Model file for the job. Use its own axes, mm. A direction names the side the tool comes from. Round coordinates to 2 decimals unless told otherwise and drop trailing zeros. Loops run counter-clockwise (first coordinate to the right, second up) from the corner with the lowest first, then second, coordinate; pieces in that order, holes last. Notation, with made-up numbers: M -31,22.5 L 2,22.5 A13 cw 2,38.5 Z; hole C 18,40.25 d2. An arc over 180 degrees is marked long. Use a Markdown table: item, result. Add a question column.
Item 1: Pin check, flat tips, straight feed: P1, Ø1, axis at x = 19.5, y = 10, coming from the -Z side; P2, Ø8.5, axis at x = -25.5, z = 47, coming from the -Y side; P3, Ø0.9, axis at x = -37.5, y = 5.5, coming from the -Z side. Stop position of each tip, or through.
Item 2: Tool access for faces 5 (the cylindrical face through (-16.14, 13.25, 51.03)), 6 (the flat face through (0, 5.25, 48)), 7 (the flat face through (-1, 16, 46)), 8 (the flat face through (-37, -2.95, 29)), 9 (the flat face through (37, 5, 21.5)): list every direction of +Z, -Z, +X, -X, +Y, -Y with a clear straight run to the whole face (end or side of a thin tool).
Item 3: Two-plate mould, pull along X, no slides. Class faces 1 (the flat face through (42, 23, 34.244)), 2 (the flat face through (43, 13, 38)), 3 (the flat face through (1, 16, 46)), 4 (the cylindrical face through (-38.19, 6.16, 17.95)): +X half, -X half, draft (parallel to the pull), parting line (faces both ways), or undercut.
Item 4: Saw through at D-D on z = 46. Give the number of separate pieces and of enclosed holes in the cut face, then the cut area to 3 significant figures.
Item 5: Saw through at C-C on x = 37. Write the cut outline in (y, z), then the cut area to 3 significant figures.
Item 6: Saw through at A-A on z = 19. Write the cut outline in (x, y), then the cut area to 3 significant figures.
Item 7: Wall check: L1, parallel to X at y = 5, z = 18; L2, parallel to Y at x = 37, z = 17.75; L3, parallel to X at y = 8, z = 27. Give the ranges that are in metal, low to high. Write a range as from..to.
Item 8: Saw through at B-B on z = 40. Write the cut outline in (x, y), then the cut area to 3 significant figures.
```python
from build123d import *

# Parameters (mm, degrees)
F0_W          = 12
F0_H          = 16.5
F0_R          = 1.6
F1_DEPTH      = 17.5
F5_W          = 12
F5_H          = 16.5
F6_DEPTH      = 3
F2_W          = 12
F2_H          = 16.4
F7_DEPTH      = 35.5
F7_DEPTH_BACK = 3
F11_W         = 50
F11_H         = 5.5
F12_DEPTH     = 90
F14_DEPTH     = 10
F15_R         = 1.5
F16_DEPTH     = 7
F17_R         = 8
F18_DEPTH     = 15
F22_R         = 8
F22_R_2       = 6
F23_DEPTH     = 6
F25_DEPTH     = 25
F26_R         = 2.25
F27_DEPTH     = 25
F28_R         = 2.25
F29_DEPTH     = 3
F30_W         = 20
F30_H         = 18.7556861639
F31_DEPTH     = 2


# Not quite as in the source:
# - a feature of the source that left no trace in its solid (it failed there, or was rolled back) is left out


with BuildPart() as f1:
    # F0 (on Top) → F1 (new body)
    with BuildSketch(Plane.XY):
        Polygon((-43, -44.5), (43, -44.5), (43, -3), (31, -3), (31, -11.5), (-31, -11.5), (-31, -3), (-43, -3), align=None)
        with Locations((37, 5.25)):
            Rectangle(F0_W, F0_H)
        with Locations((37, 5.25)):
            Circle(F0_R, mode=Mode.SUBTRACT)
        with Locations((-37, 5.25)):
            Rectangle(F0_W, F0_H)
        with Locations((-37, 5.25)):
            Circle(F0_R, mode=Mode.SUBTRACT)
        Polygon((31, 13.5), (43, 13.5), (43, 44.5), (-43, 44.5), (-43, 13.5), (-31, 13.5), (-31, 25.5), (31, 25.5), align=None)
    extrude(amount=F1_DEPTH)

    # F5 (on face) → F6 (cut)
    with BuildSketch(Plane.XY.offset(17.5)):
        with Locations((-37, 5.25)):
            Rectangle(F5_W, F5_H)
        with Locations((37, 5.25)):
            Rectangle(F5_W, F5_H)
    extrude(amount=-F6_DEPTH, mode=Mode.SUBTRACT)

    # F11 (on face) → F12 (cut)
    with BuildSketch(Plane(origin=(-43, 0, 0), x_dir=(0, -1, 0), z_dir=(-1, 0, 0))):
        with Locations((0, 2.75)):
            Rectangle(F11_W, F11_H)
    extrude(amount=-F12_DEPTH, mode=Mode.SUBTRACT)


with BuildPart() as f7:
    # F2 (on face) → F7 (new body, two sides)
    with BuildSketch(Plane.XY.offset(17.5)) as f7_sk:
        with Locations((37, 5.25)):
            Rectangle(F2_W, F2_H)
    extrude(amount=F7_DEPTH)
    extrude(f7_sk.sketch, amount=-F7_DEPTH_BACK)



with BuildPart() as f7b:
    # F2 (on face) → F7, piece 2 (new body, two sides)
    with BuildSketch(Plane.XY.offset(17.5)) as f7_2_sk:
        with Locations((-37, 5.25)):
            Rectangle(F2_W, F2_H)
    extrude(amount=F7_DEPTH)
    extrude(f7_2_sk.sketch, amount=-F7_DEPTH_BACK)


with BuildPart() as f7_1:
    add(f7.part)

    add(f7b.part)  # F14 merges F7b
    # F13 (on face) → F14 (join)
    with BuildSketch(Plane.XY.offset(53)):
        Polygon((43, -6.75), (43, 13.5), (43, 17.25), (-43, 17.25), (-43, -6.75), align=None)
    extrude(amount=-F14_DEPTH)

    # F15 (on face) → F16 (cut)
    with BuildSketch(Plane(origin=(0, 0, 14.5), x_dir=(1, 0, 0), z_dir=(0, 0, -1))):
        with Locations((-37, -5.25)):
            Circle(F15_R)
        with Locations((37, -5.25)):
            Circle(F15_R)
    extrude(amount=-F16_DEPTH, mode=Mode.SUBTRACT)

    # F17 (on face) → F18 (cut)
    with BuildSketch(Plane.XY.offset(53)):
        with Locations((16.3168814033, 5.25)):
            Circle(F17_R)
        with Locations((-16.3168814033, 5.25)):
            Circle(F17_R)
    extrude(amount=-F18_DEPTH, mode=Mode.SUBTRACT)

    # F22 (on offset) → F23 (join)
    with BuildSketch(Plane.XY.offset(49)):
        with Locations((-16.3168814033, 5.25)):
            Circle(F22_R)
        with Locations((-16.3168814033, 5.25)):
            Circle(F22_R_2, mode=Mode.SUBTRACT)
        with Locations((16.3168814033, 5.25)):
            Circle(F22_R)
        with Locations((16.3168814033, 5.25)):
            Circle(F22_R_2, mode=Mode.SUBTRACT)
    extrude(amount=-F23_DEPTH)

    # F24 (on face) → F25 (cut)
    with BuildSketch(Plane.XY.offset(53)):
        with BuildLine():
            Line((-30, 5.25), (-30, -6.75))
            Line((-30, -6.75), (30, -6.75))
            Line((30, -6.75), (30, 5.25))
            Line((30, 5.25), (-10.3168814033, 5.25))
            ThreePointArc((-10.3168814033, 5.25), (-16.3168814033, -0.75), (-22.3168814033, 5.25))
            Line((-22.3168814033, 5.25), (-30, 5.25))
        make_face()
        with BuildLine():
            ThreePointArc((-10.3168814033, 5.25), (-16.3168814033, 11.25), (-22.3168814033, 5.25))
            Line((-22.3168814033, 5.25), (-10.3168814033, 5.25))
        make_face()
        with BuildLine():
            Line((-10.3168814033, 5.25), (-22.3168814033, 5.25))
            ThreePointArc((-22.3168814033, 5.25), (-16.3168814033, -0.75), (-10.3168814033, 5.25))
        make_face()
    extrude(amount=-F25_DEPTH, mode=Mode.SUBTRACT)

    # F26 (on face) → F27 (cut)
    with BuildSketch(Plane.XZ.offset(-5.25)):
        with Locations((-4.75, 46)):
            Circle(F26_R)
        with Locations((4.75, 46)):
            Circle(F26_R)
    extrude(amount=-F27_DEPTH, mode=Mode.SUBTRACT)

    # F28 (on face) → F29 (cut)
    with BuildSketch(Plane(origin=(0, 17.25, 0), x_dir=(-1, 0, 0), z_dir=(0, 1, 0))):
        Polygon((8.5, 43.8349364905), (8.5, 48.1650635095), (4.75, 50.3301270189), (1, 48.1650635095), (1, 43.8349364905), (4.75, 41.6698729811), align=None)
        with Locations((4.75, 46)):
            Circle(F28_R, mode=Mode.SUBTRACT)
        Polygon((-1, 43.8349364905), (-1, 48.1650635095), (-4.75, 50.3301270189), (-8.5, 48.1650635095), (-8.5, 43.8349364905), (-4.75, 41.6698729811), align=None)
        with Locations((-4.75, 46)):
            Circle(F28_R, mode=Mode.SUBTRACT)
    extrude(amount=-F29_DEPTH, mode=Mode.SUBTRACT)

    # F30 (on face) → F31 (join)
    with BuildSketch(Plane.YZ.offset(43)):
        with Locations((23.45, 43.622156918)):
            Rectangle(F30_W, F30_H)
    extrude(amount=-F31_DEPTH)


solid = f7_1.part
```
Entries:
| question | item | result |
|---|---|---|
| 1 | P1 | z = 43 |
| 1 | P2 | y = 5.25 |
| 1 | P3 | z = 21.5 |
| 2 | face 5 | +Z, -Y |
| 2 | face 6 | +Z, -Z, -Y |
| 2 | face 7 | +Y |
| 2 | face 8 | -Z, +X, -X, -Y |
| 2 | face 9 | -Z |
| 3 | face 1 | draft |
| 3 | face 2 | +X half |
| 3 | face 3 | undercut |
| 3 | face 4 | undercut |
| 4 | separate pieces | 3 |
| 4 | enclosed holes | 0 |
| 4 | area | 1,140 mm2 |
| 5 | outline | M -6.75,43 L -2.95,43 L -2.95,14.5 L 3.75,14.5 L 3.75,21.5 L 6.75,21.5 L 6.75,14.5 L 13.45,14.5 L 13.45,43 L 17.25,43 L 17.25,53 L -6.75,53 Z |
| 5 | area | 686 mm2 |
| 6 | outline | M -43,-2.95 L -31,-2.95 L -31,13.45 L -43,13.45 Z; M 31,-2.95 L 43,-2.95 L 43,13.45 L 31,13.45 Z; hole C -37,5.25 d3; hole C 37,5.25 d3 |
| 6 | area | 379 mm2 |
| 7 | L1 | -43..-38.48, -35.52..-31, 31..35.52, 38.48..43 |
| 7 | L2 | -2.95..3.75, 6.75..13.45 |
| 7 | L3 | -43..-31, 31..43 |
| 8 | outline | M -43,-2.95 L -31,-2.95 L -31,13.45 L -43,13.45 Z; M 31,-2.95 L 43,-2.95 L 43,33.45 L 41,33.45 L 41,13.45 L 31,13.45 Z |
| 8 | area | 434 mm2 |
